from build123d import *

# Parameters (mm, degrees)
SKETCH_1_W          = 56
SKETCH_1_H          = 30
EXTRUDE_1_DEPTH     = 8
SKETCH_2_W          = 32
SKETCH_2_H          = 22
EXTRUDE_2_DEPTH     = 4
CUT_EXTRUDE_1_DEPTH = 60.203040462
SKETCH_4_W          = 32
SKETCH_4_H          = 8
EXTRUDE_3_DEPTH     = 8
EXTRUDE_8_DEPTH     = 13
CUT_EXTRUDE_2_DEPTH = 53.659282183
RIB_1_REACH         = 52.488
SKETCH_13_WALL_W    = 150.145150152
SKETCH_13_WALL_H    = 8


with BuildPart() as part:
    # 草图1 → 凸台-拉伸1 (new body)
    with BuildSketch(Plane(origin=(0, 0, 0), x_dir=(1, 0, 0), z_dir=(0, 1, 0))):
        Rectangle(SKETCH_1_W, SKETCH_1_H)
    extrude(amount=EXTRUDE_1_DEPTH)

    # 草图2 → 凸台-拉伸2 (add)
    with BuildSketch(Plane(origin=(0, 8, 0), x_dir=(1, 0, 0), z_dir=(0, 1, 0))):
        with Locations((-12, -4)):
            Rectangle(SKETCH_2_W, SKETCH_2_H)
    extrude(amount=EXTRUDE_2_DEPTH)

    # 草图3 → 切除-拉伸1 (cut, through all)
    with BuildSketch(Plane.ZY.offset(28)):
        Polygon((9, 0), (11.886751346, 5), (-5.886751346, 5), (-3, 0), align=None)
    extrude(amount=-CUT_EXTRUDE_1_DEPTH, mode=Mode.SUBTRACT)

    # 草图4 → 凸台-拉伸3 (add)
    with BuildSketch(Plane(origin=(0, 8, 0), x_dir=(1, 0, 0), z_dir=(0, 1, 0))):
        with Locations((-12, 11)):
            Rectangle(SKETCH_4_W, SKETCH_4_H)
    extrude(amount=EXTRUDE_3_DEPTH)

    # 草图7 → 凸台-拉伸8 (add)
    with BuildSketch(Plane(origin=(0, 0, -15), x_dir=(-1, 0, 0), z_dir=(0, 0, -1))):
        with BuildLine():
            Line((-28, 8), (-28, 21))
            ThreePointArc((-28, 21), (-16, 33), (-4, 21))
            Line((-4, 21), (-4, 8))
            Line((-4, 8), (-28, 8))
        make_face()
    extrude(amount=-EXTRUDE_8_DEPTH)

    # 草图8 → 切除-拉伸2 (cut, through all)
    with BuildSketch(Plane(origin=(0, 0, -15), x_dir=(-1, 0, 0), z_dir=(0, 0, -1))):
        with BuildLine():
            Line((-22, 18.5), (-22, 23.5))
            ThreePointArc((-22, 23.5), (-16, 29.5), (-10, 23.5))
            Line((-10, 23.5), (-10, 18.5))
            ThreePointArc((-10, 18.5), (-16, 12.5), (-22, 18.5))
        make_face()
    extrude(amount=-CUT_EXTRUDE_2_DEPTH, mode=Mode.SUBTRACT)

    # 草图13 wall → 筋1 (add, up to next)
    with BuildSketch(Plane(origin=(-6, 24.5, -11), x_dir=(0.932798134406, 0.360399279202, 0), z_dir=(-0.360399279202, 0.932798134406, 0)), mode=Mode.PRIVATE) as rib_1_sk1:
        Rectangle(SKETCH_13_WALL_W, SKETCH_13_WALL_H)
    rib_1_tool1 = extrude(rib_1_sk1.sketch, amount=-RIB_1_REACH, mode=Mode.PRIVATE) - part.part
    add(rib_1_tool1.solids().sort_by_distance((-6, 24.5, -11))[0])


solid = part.part
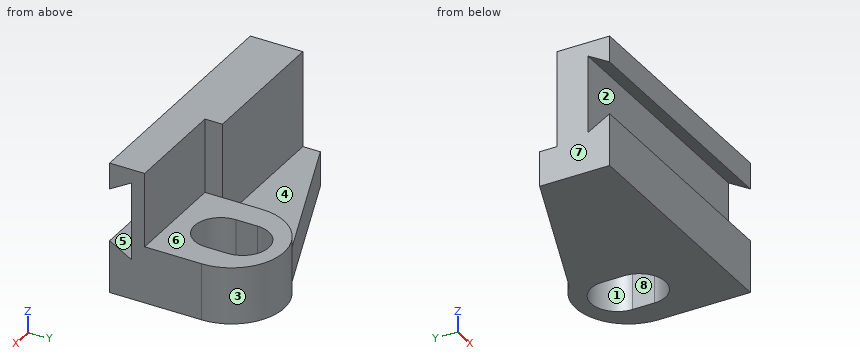
Input: part model. Units: mm. Frame: model coordinates. Face numbers are marked on the shaded views. A direction names the side the tool comes from. Give positions to 0.01 mm unless a question says otherwise; leave off trailing zeros. Write each loop counter-clockwise with the first axis right and the second up, starting at its lowest first coordinate (ties: lowest second). Pieces come first, ordered by that corner, then holes. Notation, with made-up numbers: (15, 35.25) -> (52, 35.25) arc R19 ccw to (52, 63.25) -> close; hole circle Ø2 at (-40, 68.25). An arc over 180 degrees is marked (long way). Use one line per item in the form item = value. Start each with the question number.
1) Section query D-D on y = 10. Return the cut outline in (x, z).
2) Draft query along X for the marked faces 1, 2 and 3. Return one class per face: pulls with the +X half, pulls with the -X half, needs draft (parallel to the pull), parting line crosses it, or undercut.
3) Section query C-C on y = 28. Return the cut outline in (x, z), then the cut area to 3 significant figures.
4) Pin query (flat end, axial travel): pin 1 (4 mm diameter, centred on x = -16.5, z = 3, fed in from +Y); pin 2 (1.2 mm diameter, centred on y = 11, z = 10, fed in from +X); pin 3 (2.5 mm diameter, centred on y = 17.5, z = -3.5, fed in from -X). Return the tip coordinate at first contact, or that it passes through.
5) Ray query, probe 1 along X at (y, z) = (9.5, 11.5); probe 2 along Z at (x, y) = (15.5, 32.5); probe 3 along Z at (x, y) = (-15.5, 18). Return the intervals inside material, ascending. Write a range as from..to.
6) Set-up query: the marked faces 4, 5, 6, 7 and 8. Return all of +Z, -Z, +X, -X, +Y, -Y with unobstructed straight access to the full face (end or side cutting, diameter ignored); none if empty.
7) Section query A-A on x = 16. Return the cut outline in (y, z).
8) Section query B-B on z = -13. Return the cut outline in (x, y), then the cut area to 3 significant figures.
Outcome:
q1.outline = (-28, -15) -> (28, -15) -> (28, -2) -> (4, -2) -> (4, 15) -> (-28, 15) -> close
q2.face_1 = undercut
q2.face_2 = needs draft
q2.face_3 = parting line crosses it
q3.outline = (3.06, -15) -> (12.03, -15) -> (12.03, -2) -> (6.25, -2) -> (6.25, -7) -> (3.06, -7) -> close; (19.97, -15) -> (25.75, -15) -> (25.75, -2) -> (19.97, -2) -> close
q3.area = 176 mm^2
q4.pin_1 = 12
q4.pin_2 = 4
q4.pin_3 = 4
q5.probe_1 = -28..4
q5.probe_2 = -15..-2
q5.probe_3 = -15..-7
q6.face_4 = +Z, -X, +Y
q6.face_5 = +X, -X
q6.face_6 = +Z, +X, +Y
q6.face_7 = +Z, -Z, -X, +Y, -Y
q6.face_8 = +Z, -Z
q7.outline = (0, -15) -> (12.5, -15) -> (12.5, -2) -> (8, -2) -> (8, 15) -> (0, 15) -> (0, 9) -> (5, 11.89) -> (5, -5.89) -> (0, -3) -> close; (29.5, -15) -> (33, -15) -> (33, -2) -> (29.5, -2) -> close
q8.outline = (-28, 0) -> (28, 0) -> (28, 21) arc R12 ccw to (7.93, 29.88) -> (-28, 16) -> close; hole (10, 18.5) arc R6 ccw to (22, 18.5) -> (22, 23.5) arc R6 ccw to (10, 23.5) -> close
q8.area = 1,270 mm^2
